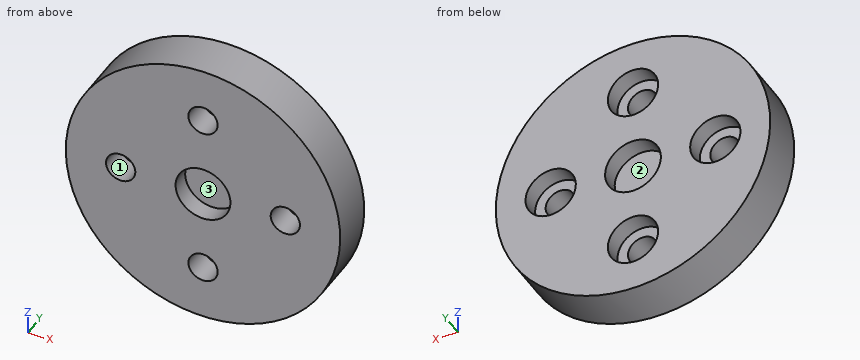
from build123d import *

# Parameters (mm, degrees)
SKETCH1_R           = 15
BOSS_EXTRUDE1_DEPTH = 5
SKETCH2_R           = 3
CUT_EXTRUDE1_DEPTH  = 2
SKETCH3_R           = 1.6
CUT_EXTRUDE2_DEPTH  = 5
SKETCH4_R           = 2.75
SKETCH4_R_2         = 3.05
CUT_EXTRUDE3_DEPTH  = 2


with BuildPart() as part:
    # Sketch1 → Boss-Extrude1 (new body)
    with BuildSketch(Plane(origin=(0, 0, 0), x_dir=(1, 0, 0), z_dir=(0, 1, 0))):
        with Locations(Location((0, 0, 0), (0, 0, 270))):
            Circle(SKETCH1_R)
    extrude(amount=BOSS_EXTRUDE1_DEPTH)

    # Sketch2 → Cut-Extrude1 (cut)
    with BuildSketch(Plane.XZ):
        with Locations(Location((0, 0, 0), (0, 0, 270))):
            Circle(SKETCH2_R)
    extrude(amount=-CUT_EXTRUDE1_DEPTH, mode=Mode.SUBTRACT)

    # Sketch3 → Cut-Extrude2 (cut)
    with BuildSketch(Plane(origin=(0, 5, 0), x_dir=(1, 0, 0), z_dir=(0, 1, 0))):
        with Locations(Location((0, 9, 0), (0, 0, 270))):
            Circle(SKETCH3_R)
        with Locations(Location((0, -9, 0), (0, 0, 270))):
            Circle(SKETCH3_R)
        with Locations(Location((9, 0, 0), (0, 0, 270))):
            Circle(SKETCH3_R)
        with Locations(Location((-9, 0, 0), (0, 0, 270))):
            Circle(SKETCH3_R)
    extrude(amount=-CUT_EXTRUDE2_DEPTH, mode=Mode.SUBTRACT)

    # Sketch4 → Cut-Extrude3 (cut)
    with BuildSketch(Plane(origin=(0, 5, 0), x_dir=(1, 0, 0), z_dir=(0, 1, 0))):
        with Locations(Location((0, 9, 0), (0, 0, 270))):
            Circle(SKETCH4_R)
        with Locations(Location((-9, 0, 0), (0, 0, 270))):
            Circle(SKETCH4_R)
        with Locations(Location((9, 0, 0), (0, 0, 270))):
            Circle(SKETCH4_R)
        with Locations(Location((0, -9, 0), (0, 0, 270))):
            Circle(SKETCH4_R)
        with Locations(Location((0, 0, 0), (0, 0, 270))):
            Circle(SKETCH4_R_2)
    extrude(amount=-CUT_EXTRUDE3_DEPTH, mode=Mode.SUBTRACT)


solid = part.part
Verification items for the finished model (mm, model axes). Face numbers are marked on the shaded views. A direction names the side the tool comes from. Round coordinates to 2 decimals unless told otherwise and drop trailing zeros. Order: outer loops, then holes, each group sorted by start corner. A loop starts at its lowest first (then second) coordinate and runs counter-clockwise, first axis right, second up. Notation, with made-up numbers: (37.25, 3) -> (64.25, 3) arc R8 ccw to (64.25, 13) -> close; hole circle Ø1 at (34.25, 6.25). An arc over 180 degrees is marked (long way). Put each result on its own line as item: value.
1) Set-up check for the marked faces 1, 2 and 3: record each of +Z, -Z, +X, -X, +Y, -Y from which the full face is reachable in a straight line by a thin tool's end or side.
Final values:
face 1: +Y, -Y
face 2: +Y
face 3: -Y
2) Section check A-A (x = -9). Record the cut outline in (y, z).
Final values:
outline: (0, -12) -> (5, -12) -> (5, -2.75) -> (3, -2.75) -> (3, -1.6) -> (0, -1.6) -> close; (0, 1.6) -> (3, 1.6) -> (3, 2.75) -> (5, 2.75) -> (5, 12) -> (0, 12) -> close
3) Section check B-B (z = 9). Record the cut outline in (x, y).
Final values:
outline: (-12, 0) -> (-1.6, 0) -> (-1.6, 3) -> (-2.75, 3) -> (-2.75, 5) -> (-12, 5) -> close; (1.6, 0) -> (12, 0) -> (12, 5) -> (2.75, 5) -> (2.75, 3) -> (1.6, 3) -> close
4) Material ranges on line 1 (X direction, y = 1.85, z = 0); line 2 (X direction, y = 3.6, z = 0); line 3 (X direction, y = 2.3, z = -1), recorded low to high.
Final values:
line 1: x = -15 to -10.6, -7.4 to -3, 3 to 7.4, 10.6 to 15
line 2: x = -15 to -11.75, -6.25 to -3.05, 3.05 to 6.25, 11.75 to 15
line 3: x = -14.97 to -10.25, -7.75 to 7.75, 10.25 to 14.97
5) Section check D-D (x = 0). Record the cut outline in (y, z), then the cut area to 3 significant figures.
Final values:
outline: (0, -15) -> (5, -15) -> (5, -11.75) -> (3, -11.75) -> (3, -10.6) -> (0, -10.6) -> close; (0, -7.4) -> (3, -7.4) -> (3, -6.25) -> (5, -6.25) -> (5, -3.05) -> (3, -3.05) -> (3, 3.05) -> (5, 3.05) -> (5, 6.25) -> (3, 6.25) -> (3, 7.4) -> (0, 7.4) -> (0, 3) -> (2, 3) -> (2, -3) -> (0, -3) -> close; (0, 10.6) -> (3, 10.6) -> (3, 11.75) -> (5, 11.75) -> (5, 15) -> (0, 15) -> close
area: 84.6 mm^2
6) Section check C-C (y = 2.65). Record the cut outline in (x, z), then the cut area to 3 significant figures.
Final values:
outline: circle Ø30 at (0, 0); hole circle Ø3.2 at (-9, 0); hole circle Ø3.2 at (0, -9); hole circle Ø3.2 at (0, 9); hole circle Ø3.2 at (9, 0)
area: 675 mm^2
7) Depth check by flat-ended pin: pin 1 (5 mm diameter, centred on x = 0, z = 9, fed in from +Y). Enter the tip coordinate at first touch or a pass-through.
Final values:
pin 1: stops at y = 3
